Could you check a few things on this model? Use its own coordinates, in mm. A direction names the side the tool comes from. Round coordinates to 2 decimals unless told otherwise and drop trailing zeros. Loops run counter-clockwise (first coordinate to the right, second up) from the corner with the lowest first, then second, coordinate; pieces in that order, holes last. Notation, with made-up numbers: (37.5, 86.25) -> (47.5, 86.25) arc R28 cw to (47.5, 104.25) -> close; hole circle Ø11 at (52, 70). An arc over 180 degrees is marked (long way). One line per item, written item: value.
Solid Edge part; units mm, degrees
sketch "Sketch1" plane through (0, 0, 0) normal (0, -1, 0) x (1, 0, 0)
  circle A0 centre (0, 0) radius 5.15
  line L0 (-12, -5.2) -> (12, -5.2)
  line L1 (12, -5.2) -> (12, -3.2)
  line L2 (12, -3.2) -> (7, -3.2)
  line L3 (7, -3.2) -> (7, 0)
  arc A1 (7, 0) -> (-7, 0) centre (0, 0) ccw
  line L4 (-7, 0) -> (-7, -3.2)
  line L5 (-12, -3.2) -> (-7, -3.2)
  line L6 (-12, -5.2) -> (-12, -3.2)
  dimension "D1" = 12
  dimension "D2" = 12
  dimension "D3" = 12
extrude "Protrusion1" add sketch "Sketch1" along normal mid plane 6
hole "Hole1" at (-9.5, 0, -3.2) direction (0, 0, -1) diameter 3.3 end up to next
hole "Hole2" at (9.5, 0, -3.2) direction (0, 0, -1) diameter 3.3 end up to next
sketch "Sketch2" plane through (9.5, 0, -3.2) normal (0, 0, 1) x (-1, 0, 0)
  circle A0 centre (19, 0) radius 2.75
  circle A1 centre (0, 0) radius 2.75
extrude "Cutout1" cut sketch "Sketch2" along normal up to next
properties material "ABS, alto impacto"
(1) Imagine slicing it at C-C on z = -3.5. Write out the boundary of the cut face in (x, y), then the cut area to 3 significant figures.
Results below:
outline: (-12, -3) -> (-3.78, -3) -> (-3.78, 3) -> (-12, 3) -> close; (3.78, -3) -> (12, -3) -> (12, 3) -> (3.78, 3) -> close; hole circle Ø3.3 at (-9.5, 0); hole circle Ø3.3 at (9.5, 0)
area: 81.6 mm²
(2) For pin 1 Ø2.5 at (x, y) = (9, -1.5) entering from +Z; pin 2 Ø0.6 at (y, z) = (-2, -1) entering from +X; pin 3 Ø0.6 at (y, z) = (-2, -1.5) entering from -X, each with a flat end and sliding along its axis, tell me the tip position at first contact or that it passes through.
Results below:
pin 1: stops at z = -3.2
pin 2: stops at x = 7
pin 3: stops at x = -7
(3) Imagine slicing it at D-D on y = -2.5. Write out the boundary of the cut face in (x, z), then the cut area to 3 significant figures.
Results below:
outline: (-12, -5.2) -> (12, -5.2) -> (12, -3.2) -> (7, -3.2) -> (7, 0) arc R7 ccw to (-7, 0) -> (-7, -3.2) -> (-12, -3.2) -> close; hole circle Ø10.3 at (0, 0)
area: 86.4 mm²
(4) On a 3-axis mill with a long thin cutter (end or side, diameter ignored), from which of +Z, -Z, +X, -X, +Y, -Y can I reach the whole of each face in a straight line? I mean faces 5 (the face through (-6.75, 0.02, -0.71)), 6 (the face through (7, 2, -2)), 7 (the face through (6.75, -0.02, -0.71)), 8 (the face through (-7, -2, -2)). Say none if no direction works.
Results below:
face 5: +Z, -X
face 6: +Z, +X, +Y, -Y
face 7: +Z, +X
face 8: +Z, -X, +Y, -Y
(5) Imagine slicing it at A-A on y = 0. Write out the boundary of the cut face in (x, z).
Results below:
outline: (-12, -5.2) -> (-11.15, -5.2) -> (-11.15, -3.2) -> (-12, -3.2) -> close; (-7.85, -5.2) -> (7.85, -5.2) -> (7.85, -3.2) -> (6.75, -3.2) -> (6.75, 1.85) arc R7 ccw to (-6.75, 1.85) -> (-6.75, -3.2) -> (-7.85, -3.2) -> close; (11.15, -5.2) -> (12, -5.2) -> (12, -3.2) -> (11.15, -3.2) -> close; hole circle Ø10.3 at (0, 0)
(6) Imagine slicing it at B-B on x = 9.5. Write out the boundary of the cut face in (y, z).
Results below:
outline: (-3, -5.2) -> (-1.65, -5.2) -> (-1.65, -3.2) -> (-3, -3.2) -> close; (1.65, -5.2) -> (3, -5.2) -> (3, -3.2) -> (1.65, -3.2) -> close
(7) We'd pull the mould along X, two halves only. Please class faces 1 (the face through (7, -2, -2)), 2 (the face through (7.9, 0.4, -4.2)), 3 (the face through (-11.1, 0.4, -4.2)), 4 (the face through (-2, -3, -5)): +X half, -X half, draft (parallel to the pull), parting line (faces both ways), or undercut.
Results below:
face 1: +X half
face 2: undercut
face 3: undercut
face 4: draft
(8) Please list where these lines run through material, in increasing order: L1, parallel to X at y = 0, z = -4.4; L2, parallel to Y at x = -9.5, z = -4.25; L3, parallel to X at y = 0, z = -4.
Results below:
L1: x = -12 to -11.15, -7.85 to -2.68, 2.68 to 7.85, 11.15 to 12
L2: y = -3 to -1.65, 1.65 to 3
L3: x = -12 to -11.15, -7.85 to -3.24, 3.24 to 7.85, 11.15 to 12
